from build123d import *

# Parameters (mm, degrees)
SKETCH1_R           = 3.937
SKETCH1_R_2         = 2.54
BOSS_EXTRUDE1_DEPTH = 0.762
FILLET1_R           = 1.778
FILLET2_R           = 7.62


with BuildPart() as part:
    # Sketch1 → Boss-Extrude1 (new, symmetric)
    with BuildSketch(Plane(origin=(0, 0, 0), x_dir=(0, 0, -1), z_dir=(1, 0, 0))):
        with BuildLine():
            Line((-0.16671433, 27.427788703), (-7.62, 27.051))
            Line((-7.62, 27.051), (-24.562678082, 42.265364279))
            ThreePointArc((-24.562678082, 42.265364279), (-26.249752812, 49.261680344), (-20.32, 53.34))
            Line((-20.32, 53.34), (10.16, 53.34))
            Line((10.16, 53.34), (10.16, 36.49278302))
            ThreePointArc((10.16, 36.49278302), (15.447327881, 28.30660931), (15.005535214, 18.571410526))
            Line((15.005535214, 18.571410526), (7.145492959, -2.646947368))
            ThreePointArc((7.145492959, -2.646947368), (-3.137043416, -6.94430404), (-6.709547814, 3.611975654))
            Line((-6.709547814, 3.611975654), (2.391547814, 20.518024346))
            ThreePointArc((2.391547814, 20.518024346), (3.070881997, 22.267522395), (3.302, 24.13))
            ThreePointArc((3.302, 24.13), (2.275160794, 26.523083233), (-0.16671433, 27.427788703))
        make_face()
        with Locations(Location((0, 0, 0), (0, 0, 180))):
            Circle(SKETCH1_R, mode=Mode.SUBTRACT)
        with Locations(Location((-20.32, 46.99, 0), (0, 0, 180))):
            Circle(SKETCH1_R_2, mode=Mode.SUBTRACT)
    extrude(amount=BOSS_EXTRUDE1_DEPTH, both=True)

    # Fillet1
    fillet1_edges = [part.edges().sort_by_distance(p)[0] for p in [
        (0, 27.051, 7.62),
        (0, 53.34, -10.16),
    ]]
    fillet(fillet1_edges, radius=FILLET1_R)

    # Fillet2
    fillet2_edges = [part.edges().sort_by_distance(p)[0] for p in [
        (0, 36.49278302, -10.16),
    ]]
    fillet(fillet2_edges, radius=FILLET2_R)


solid = part.part
Part model, mm, in its own coordinate system. A direction names the side the tool comes from. Coordinates: 2 decimals unless noted, no trailing zeros. Loops run counter-clockwise (first coordinate to the right, second up) from the corner with the lowest first, then second, coordinate; pieces in that order, holes last. Notation, with made-up numbers: (33, 67.25) - (45, 67.25) arc R15 ccw to (45, 81.25) - close; hole circle Ø5 at (51.5, -1). An arc over 180 degrees is marked (long way). Write each question's results on one line, items separated by ' | '. Start each with the question number.
Q1. Drop a flat-ended pin along its axis: pin 1 Ø12.5 at (y, z) = (0, 0) entering from +X. Give the stop position or say it passes through.
Q2. Which spindle directions (+Z, -Z, +X, -X, +Y, -Y) get a long thin tool onto all of the face, cutting with end or side? Do faces 1 (the flat face through (0.01, 27.26, 3.48)), 2 (the flat face through (0.01, 11.95, 2.22)), 3 (the cylindrical face through (-0.01, 52.81, -9.65)). Say none if no direction does.
Q3. Slice it at B-B on y = 46.99. Give the cut face in (x, z).
Q4. Two-plate mould, pull along Y, no slides. Class faces 4 (the cylindrical face through (0, 26.5, -2.3)), 5 (the cylindrical face through (0.011, 27.144, -15.716)), 6 (the cylindrical face through (-0.011, 37.039, -10.633)), 7 (the flat face through (0, 46, -10.16)): +Y half, -Y half, draft (parallel to the pull), parting line (faces both ways), or undercut.
Q5. Slice it at A-A on x = 0.2. Give the cut face in (y, z), and give its area (3 significant figures).
Q6. Probe line 1 along Z through (x, y) = (-0.15, 46.99); line 2 along Y through (x, z) = (-0.1, 1); line 3 along Y through (x, z) = (0, 20.32). List the from-to ranges inside material, lowest first.
Q7. Slice it at C-C on z = 2. Give the cut face in (x, y).
Q8. Slice it at D-D on z = 18.5. Give the cut face in (x, y), and give its area (3 significant figures).
Answer:
1) pin 1: stops at x = 0.76
2) face 1: +X, -X | face 2: +Z, +X, -X | face 3: -Z, +X, -X, +Y
3) outline: (-0.76, -10.16) - (0.76, -10.16) - (0.76, 17.78) - (-0.76, 17.78) - close; (-0.76, 22.86) - (0.76, 22.86) - (0.76, 26.67) - (-0.76, 26.67) - close
4) face 4: undercut | face 5: parting line | face 6: +Y half | face 7: draft
5) outline: (-2.65, -7.15) - (18.57, -15.01) arc R16 ccw to (34.67, -12.04) arc R7.62 cw to (39.68, -10.16) - (51.56, -10.16) arc R1.78 ccw to (53.34, -8.38) - (53.34, 20.32) arc R6.35 ccw to (42.27, 24.56) - (27.54, 8.17) arc R1.78 ccw to (27.09, 6.89) - (27.43, 0.17) arc R3.3 cw to (24.13, -3.3) arc R7.62 cw to (20.52, -2.39) - (3.61, 6.71) arc R7.62 ccw (long way) to start; hole circle Ø7.87 at (0, 0); hole circle Ø5.08 at (46.99, 20.32) | area: 1,240 mm2
6) line 1: z = -10.16 to 17.78, 22.86 to 26.67 | line 2: y = -7.55 to -3.81, 3.81 to 14.22, 27.39 to 53.34 | line 3: y = 38.46 to 44.45, 49.53 to 53.34
7) outline: (-0.76, -7.35) - (0.76, -7.35) - (0.76, -3.39) - (-0.76, -3.39) - close; (-0.76, 3.39) - (0.76, 3.39) - (0.76, 12.36) - (-0.76, 12.36) - close; (-0.76, 27.34) - (0.76, 27.34) - (0.76, 53.34) - (-0.76, 53.34) - close
8) outline: (-0.76, 36.82) - (0.76, 36.82) - (0.76, 45.22) - (-0.76, 45.22) - close; (-0.76, 48.76) - (0.76, 48.76) - (0.76, 53.34) - (-0.76, 53.34) - close | area: 19.8 mm2
